Part model, mm, in its own coordinate system. A direction names the side the tool comes from. Coordinates: 2 decimals unless noted, no trailing zeros. Order: outer loops, then holes, each group sorted by start corner. A loop starts at its lowest first (then second) coordinate and runs counter-clockwise, first axis right, second up.
```python
from build123d import *

# Parameters (mm, degrees)
BOSS_EXTRUDE1_DEPTH              = 5
SKETCH2_W                        = 15
SKETCH2_H                        = 18
BOSS_EXTRUDE2_DEPTH              = 7
SKETCH3_R                        = 4.5
CUT_EXTRUDE2_DEPTH               = 4
TAP_DRILL_FOR_M8X1_25_TAP1_D     = 6.8
TAP_DRILL_FOR_M8X1_25_TAP1_DEPTH = 8


with BuildPart() as part:
    # Sketch1 → Boss-Extrude1 (new body)
    with BuildSketch(Plane(origin=(0, 0, 0), x_dir=(1, 0, 0), z_dir=(0, 1, 0))):
        with BuildLine():
            Line((0, 0), (0, 21.542378969))
            Line((0, 21.542378969), (55, 21.542378969))
            Line((55, 21.542378969), (55, 0))
            ThreePointArc((55, 0), (27.5, 2.542378969), (0, 0))
        make_face()
    extrude(amount=BOSS_EXTRUDE1_DEPTH)

    # Sketch2 → Boss-Extrude2 (add)
    with BuildSketch(Plane(origin=(0, 5, 0), x_dir=(1, 0, 0), z_dir=(0, 1, 0))):
        with Locations((27.5, 12.542378969)):
            Rectangle(SKETCH2_W, SKETCH2_H)
    extrude(amount=BOSS_EXTRUDE2_DEPTH)

    # Sketch3 → Cut-Extrude2 (cut)
    with BuildSketch(Plane(origin=(0, 0, -21.542378969), x_dir=(-1, 0, 0), z_dir=(0, 0, -1))):
        with Locations((-27.5, 6.5)):
            Circle(SKETCH3_R)
    extrude(amount=-CUT_EXTRUDE2_DEPTH, mode=Mode.SUBTRACT)

    # Tap Drill for M8x1.25 Tap1
    with Locations(Plane(origin=(0, 0, -17.542378969), x_dir=(-1, 0, 0), z_dir=(0, 0, -1))):
        with Locations((-27.5, 6.5)):
            Hole(TAP_DRILL_FOR_M8X1_25_TAP1_D / 2, depth=TAP_DRILL_FOR_M8X1_25_TAP1_DEPTH)


solid = part.part
```
(1) Tool access for faces 1 (the face through (29, 10, -17.542)), 2 (the face through (27, 8, -3.542)), 3 (the face through (20, 8, -12)), 4 (the face through (35, 8, -12)): list every direction of +Z, -Z, +X, -X, +Y, -Y with a clear straight run to the whole face (end or side of a thin tool).
(2) Drop flat-ended pins along their axis: pin 1 (1.5 mm diameter, centred on x = 10.5, z = -18.5, fed in from +Y); pin 2 (1 mm diameter, centred on x = 7.5, y = 5, fed in from +Z); pin 3 (3 mm diameter, centred on x = 24.5, y = 4, fed in from +Z); pin 4 (1 mm diameter, centred on x = 40.5, y = 6, fed in from -Z). Give the stop position or say it passes through.
(3) Slice it at C-C, the plane y = 6.5. Give the cut face in (x, z), then the cut area to 3 significant figures.
(4) Slice it at D-D, the plane x = 27.5. Give the cut face in (y, z).
(5) Probe line 1 (Y direction, x = 27.5, z = -19.3); line 2 (Y direction, x = 27.5, z = -11.75); line 3 (Y direction, x = 47, z = -12.25). List the from-to ranges inside material, lowest first.
(6) Slice it at B-B, the plane z = -9. Give the cut face in (x, y).
(7) Slice it at A-A, the plane z = -16. Give the cut face in (x, y).
Here are the results:
1. face 1: -Z
1. face 2: +Z, +X, -X, +Y
1. face 3: +Z, -Z, -X, +Y
1. face 4: +Z, -Z, +X, +Y
2. pin 1: stops at y = 5
2. pin 2: stops at z = -1.13
2. pin 3: stops at z = -2.47
2. pin 4: passes through
3. outline: (20, -21.54) - (23, -21.54) - (23, -17.54) - (24.1, -17.54) - (24.1, -9.54) - (30.9, -9.54) - (30.9, -17.54) - (32, -17.54) - (32, -21.54) - (35, -21.54) - (35, -3.54) - (20, -3.54) - close
3. area: 180 mm2
4. outline: (0, -21.54) - (2, -21.54) - (2, -17.54) - (3.1, -17.54) - (3.1, -9.54) - (9.9, -9.54) - (9.9, -17.54) - (11, -17.54) - (11, -21.54) - (12, -21.54) - (12, -3.54) - (5, -3.54) - (5, -2.54) - (0, -2.54) - close
5. line 1: y = 0 to 2, 11 to 12
5. line 2: y = 0 to 3.1, 9.9 to 12
5. line 3: y = 0 to 5
6. outline: (0, 0) - (55, 0) - (55, 5) - (35, 5) - (35, 12) - (20, 12) - (20, 5) - (0, 5) - close
7. outline: (0, 0) - (55, 0) - (55, 5) - (35, 5) - (35, 12) - (20, 12) - (20, 5) - (0, 5) - close; hole circle Ø6.8 at (27.5, 6.5)
